Autodesk Inventor part; units mm, degrees
ref_plane "YZ Plane" through (0, 0, 0) normal (1, 0, 0) x (0, 1, 0)
ref_plane "XZ Plane" through (0, 0, 0) normal (0, 1, 0) x (-1, 0, 0)
ref_plane "XY Plane" through (0, 0, 0) normal (0, 0, 1) x (1, 0, 0)
sketch "Sketch1" plane through (0, 0, 0) normal (0, 0, 1) x (1, 0, 0)
  line L0 (-30, 17.5) -> (30, 17.5)
  line L1 (30, 17.5) -> (30, -17.5)
  line L2 (30, -17.5) -> (-30, -17.5)
  line L3 (-30, -17.5) -> (-30, 17.5)
  line L4 (-2.5, 7.75) -> (25, 7.75)
  line L5 (25, 7.75) -> (25, -7.75)
  line L6 (25, -7.75) -> (-2.5, -7.75)
  line L7 (-2.5, -7.75) -> (-2.5, 7.75)
  line L8 (-14.5, 8.5) -> (-9.5, 8.5)
  line L9 (-9.5, 8.5) -> (-9.5, -8.5)
  line L10 (-9.5, -8.5) -> (-14.5, -8.5)
  line L11 (-14.5, -8.5) -> (-14.5, 8.5)
  point P0 (0, 0)
  dimension "length" = 60
  dimension "width" = 35
  dimension "d2" = 17.5
  dimension "d3" = 30
  dimension "d4" = 27.5
  dimension "d5" = 15.5
  dimension "d6" = 7.75
  dimension "d7" = 5
  dimension "d8" = 5
  dimension "d9" = 17
  dimension "d10" = 8.5
  dimension "d11" = 7
extrude "Extrusion1" add sketch "Sketch1" along normal blind 3
sketch "Sketch2" plane through (0, 0, 3) normal (0, 0, 1) x (1, 0, 0)
  line L0 (-22, 9) -> (22, 9)
  line L1 (22, 9) -> (22, -9)
  line L2 (22, -9) -> (-22, -9)
  line L3 (-22, -9) -> (-22, 9)
  line L4 (25, 7.75) -> (25, -7.75)
  line L5 (25, -7.75) -> (-2.5, -7.75)
  line L6 (-2.5, -7.75) -> (-2.5, 7.75)
  line L7 (-2.5, 7.75) -> (25, 7.75)
  line L8 (-9.5, 8.5) -> (-9.5, -8.5)
  line L9 (-9.5, -8.5) -> (-14.5, -8.5)
  line L10 (-14.5, -8.5) -> (-14.5, 8.5)
  line L11 (-14.5, 8.5) -> (-9.5, 8.5)
  line L12 (30, 17.5) -> (-30, 17.5)
  line L13 (-30, 17.5) -> (-30, -17.5)
  line L14 (-30, -17.5) -> (30, -17.5)
  line L15 (30, -17.5) -> (30, 17.5)
  point P0 (0, 0)
  dimension "d14" = 44
  dimension "d15" = 18
  dimension "d16" = 9
extrude "Extrusion2" add sketch "Sketch2" along normal blind 5 contours L7 L4 L5 L1 | L15 L14 L13 L12
hole "Hole1" at (-26, 13, 0) direction (0, 0, 1) diameter 3 end through all
pattern_linear "Rectangular Pattern1" count 2 spacing 52 along (1, 0, 0) count 2 spacing 26 along (0, -1, 0) of "Hole1"
sketch "Sketch3" plane through (0, 0, 3) normal (0, 0, -1) x (-1, 0, 0)
  line L0 (-25, -7.75) -> (-22, -7.75)
  line L1 (-22, -7.75) -> (-22, 7.75)
  line L2 (-22, 7.75) -> (-25, 7.75)
  line L3 (-25, 7.75) -> (-25, -7.75)
  point P0 (0, 0)
extrude "Extrusion3" cut sketch "Sketch3" against normal through all
sketch "Sketch4" plane through (-22, 9, 3) normal (0, -1, 0) x (1, 0, 0)
  line L0 (44, 0) -> (0, 0)
  line L1 (44, 0) -> (44, 5)
  line L2 (0, 5) -> (44, 5)
  line L3 (0, 0) -> (0, 5)
  point P0 (22, -3)
extrude "Extrusion4" cut sketch "Sketch4" against normal blind 5
sketch "Sketch5" plane through (-22, -9, 3) normal (0, 1, 0) x (1, 0, 0)
  line L0 (0, 0) -> (44, 0)
  line L1 (0, 0) -> (0, -5)
  line L2 (44, -5) -> (0, -5)
  line L3 (44, 0) -> (44, -5)
  point P0 (22, 3)
extrude "Extrusion5" cut sketch "Sketch5" against normal blind 5
properties part number "suport releu"
Can you work these out from the model? Positions are in its coordinate system, mm. A direction names the side the tool comes from. Coordinates: 2 decimals unless noted, no trailing zeros. Write each loop counter-clockwise with the first axis right and the second up, starting at its lowest first coordinate (ties: lowest second). Pieces come first, ordered by that corner, then holes. Notation, with made-up numbers: (12.5, -35.75) -> (28.5, -35.75) arc R14 cw to (28.5, -13.75) -> close; hole circle Ø2 at (16, 49.25). An arc over 180 degrees is marked (long way). Write each question's results on one line, items separated by ' | '. Start each with the question number.
Q1. I'm going to push flat-ended pins straight in: pin 1 (14 mm diameter, centred on x = 5, y = 2.5, fed in from +Z); pin 2 (2.5 mm diameter, centred on x = -26, y = -13, fed in from -Z). Where does each tip first touch, or does it pass through?
Q2. Imagine slicing it at D-D (x = 18.5). Write out the boundary of the cut face in (y, z), then the cut area to 3 significant figures.
Q3. We'd pull the mould along X, two halves only. Please class faces 4 (the face through (30, 0, 4)), 5 (the face through (-30, 0, 4)), 6 (the face through (-2.5, 0, 1)): +X half, -X half, draft (parallel to the pull), parting line (faces both ways), or undercut.
Q4. Imagine slicing it at C-C (z = 1.5). Write out the boundary of the cut face in (x, y).
Q5. Imagine slicing it at B-B (x = 26). Write out the boundary of the cut face in (y, z), then the cut area to 3 significant figures.
Q6. On a 3-axis mill with a long thin cutter (end or side, diameter ignored), from which of +Z, -Z, +X, -X, +Y, -Y can I reach the whole of each face in a straight line? I mean faces 1 (the face through (22, 11, 5)), 2 (the face through (0, -15, 8)), 3 (the face through (-9.5, 0, 1)). Say none if no direction works.
Q7. Imagine slicing it at A-A (y = 13). Write out the boundary of the cut face in (x, z), then the cut area to 3 significant figures.
Q8. If I drill on probe 1 along Y at (x, z) = (26, 7.75); probe 2 along X at (y, z) = (13, 2.25); probe 3 along X at (y, z) = (13, 3.5), over which ranges is the centre line in solid material (lowest first)?
Taken from the geometry:
1) pin 1: stops at z = 3 | pin 2: passes through
2) outline: (-17.5, 0) -> (-7.75, 0) -> (-7.75, 3) -> (-14, 3) -> (-14, 8) -> (-17.5, 8) -> close; (7.75, 0) -> (17.5, 0) -> (17.5, 8) -> (14, 8) -> (14, 3) -> (7.75, 3) -> close | area: 93.5 mm^2
3) face 4: +X half | face 5: -X half | face 6: undercut
4) outline: (-30, -17.5) -> (30, -17.5) -> (30, 17.5) -> (-30, 17.5) -> close; hole circle Ø3 at (-26, -13); hole circle Ø3 at (-26, 13); hole (-14.5, -8.5) -> (-9.5, -8.5) -> (-9.5, 8.5) -> (-14.5, 8.5) -> close; hole (-2.5, -7.75) -> (25, -7.75) -> (25, 7.75) -> (-2.5, 7.75) -> close; hole circle Ø3 at (26, -13); hole circle Ø3 at (26, 13)
5) outline: (-17.5, 0) -> (-14.5, 0) -> (-14.5, 8) -> (-17.5, 8) -> close; (-11.5, 0) -> (11.5, 0) -> (11.5, 8) -> (-11.5, 8) -> close; (14.5, 0) -> (17.5, 0) -> (17.5, 8) -> (14.5, 8) -> close | area: 232 mm^2
6) face 1: +Z | face 2: +Z, +X, -X, +Y, -Y | face 3: +Z, -Z
7) outline: (-30, 0) -> (-27.5, 0) -> (-27.5, 8) -> (-30, 8) -> close; (-24.5, 0) -> (24.5, 0) -> (24.5, 8) -> (22, 8) -> (22, 3) -> (-22, 3) -> (-22, 8) -> (-24.5, 8) -> close; (27.5, 0) -> (30, 0) -> (30, 8) -> (27.5, 8) -> close | area: 212 mm^2
8) probe 1: y = -17.5 to -14.5, -11.5 to 11.5, 14.5 to 17.5 | probe 2: x = -30 to -27.5, -24.5 to 24.5, 27.5 to 30 | probe 3: x = -30 to -27.5, -24.5 to -22, 22 to 24.5, 27.5 to 30
